```python
from build123d import *

# Parameters (mm, degrees)
EXTRUDE_1_DEPTH     = 20
CHAMFER_1_SIZE      = 10
CUT_EXTRUDE_1_DEPTH = 15
SKETCH_3_R          = 15
CUT_EXTRUDE_2_DEPTH = 20
SKETCH_4_R          = 2.25
SKETCH_4_R_2        = 10
CUT_EXTRUDE_3_DEPTH = 20
SKETCH_5_R          = 4
EXTRUDE_3_DEPTH     = 5
FILLET_1_R          = 5
SKETCH_6_R          = 1
CUT_EXTRUDE_4_DEPTH = 10
FILLET_2_R          = 5
CUT_EXTRUDE_5_REACH = 22
EXTRUDE_4_DEPTH     = 13
CUT_EXTRUDE_6_DEPTH = 5


with BuildPart() as part:
    # 스케치1 → 보스-돌출1 (new body)
    with BuildSketch(Plane.XY):
        with BuildLine():
            Line((0, 35), (40, 35))
            ThreePointArc((40, 35), (57.364817767, 36.519224699), (74.202014333, 41.030737921))
            Line((74.202014333, 41.030737921), (83.59894054, 44.450939355))
            ThreePointArc((83.59894054, 44.450939355), (128.458887284, 23.532402644), (107.540350573, -21.3275441))
            Line((107.540350573, -21.3275441), (98.143424365, -24.747745534))
            ThreePointArc((98.143424365, -24.747745534), (69.520190203, -32.417318012), (40, -35))
            Line((40, -35), (0, -35))
            ThreePointArc((0, -35), (-35, 0), (0, 35))
        make_face()
    extrude(amount=EXTRUDE_1_DEPTH)

    # 모따기1
    chamfer_1_edges = [part.edges().sort_by_distance(p)[0] for p in [
        (128.458887284, 23.532402644, 20),
        (78.900477436, 42.740838638, 20),
        (57.364817767, 36.519224699, 20),
        (20, 35, 20),
        (-35, 0, 20),
        (20, -35, 20),
        (69.520190203, -32.417318012, 20),
        (102.841887469, -23.037644817, 20),
    ]]
    chamfer(chamfer_1_edges, length=CHAMFER_1_SIZE)

    # 스케치2 → 컷-돌출1 (cut)
    with BuildSketch(Plane.XY.offset(20)):
        with BuildLine():
            Line((40, 25), (0, 25))
            ThreePointArc((0, 25), (-25, 0), (0, -25))
            Line((0, -25), (40, -25))
            ThreePointArc((40, -25), (67.783708427, -22.569240482), (94.723222932, -15.350819326))
            Line((94.723222932, -15.350819326), (104.12014914, -11.930617892))
            ThreePointArc((104.12014914, -11.930617892), (119.061961076, 20.11220121), (87.019141974, 35.054013147))
            Line((87.019141974, 35.054013147), (77.622215766, 31.633811714))
            ThreePointArc((77.622215766, 31.633811714), (59.101299543, 26.671147169), (40, 25))
        make_face()
    extrude(amount=-CUT_EXTRUDE_1_DEPTH, mode=Mode.SUBTRACT)

    # 스케치3 → 컷-돌출2 (cut)
    with BuildSketch(Plane.XY.offset(5)):
        with Locations((95.569645557, 11.561697627)):
            Circle(SKETCH_3_R)
    extrude(amount=-CUT_EXTRUDE_2_DEPTH, mode=Mode.SUBTRACT)

    # 스케치4 → 컷-돌출3 (cut)
    with BuildSketch(Plane.XY.offset(5)):
        with Locations((-10.606601718, 10.606601718)):
            Circle(SKETCH_4_R)
        with Locations((10.606601718, 10.606601718)):
            Circle(SKETCH_4_R)
        with Locations((10.606601718, -10.606601718)):
            Circle(SKETCH_4_R)
        with Locations((-10.606601718, -10.606601718)):
            Circle(SKETCH_4_R)
        Circle(SKETCH_4_R_2)
    extrude(amount=-CUT_EXTRUDE_3_DEPTH, mode=Mode.SUBTRACT)

    # 스케치5 → 보스-돌출3 (add)
    with BuildSketch(Plane.XY.offset(5)):
        with Locations((-22, 0)):
            Circle(SKETCH_5_R)
        with Locations((116.242883214, 19.08614078)):
            Circle(SKETCH_5_R)
        with Locations((59.622244076, 23.71672391)):
            Circle(SKETCH_5_R)
        with Locations((67.262763894, -19.614817223)):
            Circle(SKETCH_5_R)
    extrude(amount=EXTRUDE_3_DEPTH)

    # 필렛1
    fillet_1_edges = [part.edges().sort_by_distance(p)[0] for p in [
        (-24.840909091, -2.81588983, 7.5),
        (-24.840909091, 2.81588983, 7.5),
        (117.94937348, 22.703859809, 7.5),
        (119.875555567, 17.41171802, 7.5),
        (61.666476802, 27.154908396, 7.5),
        (56.525365318, 26.248391731, 7.5),
        (70.410078123, -22.083503744, 7.5),
        (65.149596455, -23.011068594, 7.5),
    ]]
    fillet(fillet_1_edges, radius=FILLET_1_R)

    # 스케치6 → 컷-돌출4 (cut)
    with BuildSketch(Plane.XY.offset(10)):
        with Locations((59.622244076, 23.71672391)):
            Circle(SKETCH_6_R)
        with Locations((67.262763894, -19.614817223)):
            Circle(SKETCH_6_R)
        with Locations((-22, 0)):
            Circle(SKETCH_6_R)
        with Locations((116.242883214, 19.08614078)):
            Circle(SKETCH_6_R)
    extrude(amount=-CUT_EXTRUDE_4_DEPTH, mode=Mode.SUBTRACT)

    # 필렛2
    fillet_2_edges = [part.edges().sort_by_distance(p)[0] for p in [
        (128.458887284, 23.532402644, 10),
        (78.900477436, 42.740838638, 10),
        (102.841887469, -23.037644817, 10),
        (57.364817767, 36.519224699, 10),
        (69.520190203, -32.417318012, 10),
        (20, 35, 10),
        (20, -35, 10),
        (-35, 0, 10),
    ]]
    fillet(fillet_2_edges, radius=FILLET_2_R)

    # 스케치8 → 컷-돌출5 (cut, up to next)
    with BuildSketch(Plane(origin=(0, 0, 0), x_dir=(-1, 0, 0), z_dir=(0, 0, -1)), mode=Mode.PRIVATE) as cut_extrude_5_sk1:
        with BuildLine():
            ThreePointArc((-79.499955315, -7.589413451), (-72.077330037, 3.011194044), (-70.949451732, 15.902902069))
            ThreePointArc((-70.949451732, 15.902902069), (-73.845591558, 17.930801007), (-75.873490497, 15.03466118))
            ThreePointArc((-75.873490497, 15.03466118), (-76.775793141, 4.721294761), (-82.713893363, -3.759191235))
            ThreePointArc((-82.713893363, -3.759191235), (-83.022035447, -7.281271367), (-79.499955315, -7.589413451))
        make_face()
    cut_extrude_5_tool1 = extrude(cut_extrude_5_sk1.sketch, amount=-CUT_EXTRUDE_5_REACH, mode=Mode.PRIVATE) & part.part
    add(cut_extrude_5_tool1.solids().sort_by_distance((75.648018, 4.310818, 0))[0], mode=Mode.SUBTRACT)

    # 스케치9 → 보스-돌출4 (add)
    with BuildSketch(Plane(origin=(0, 0, 20), x_dir=(-1, 0, 0), z_dir=(0, 0, -1))):
        with BuildLine():
            Line((-107.540350573, -21.3275441), (-98.143424365, -24.747745534))
            ThreePointArc((-98.143424365, -24.747745534), (-69.520190203, -32.417318012), (-40, -35))
            Line((-40, -35), (0, -35))
            ThreePointArc((0, -35), (35, 0), (0, 35))
            Line((0, 35), (-40, 35))
            ThreePointArc((-40, 35), (-57.364817767, 36.519224699), (-74.202014333, 41.030737921))
            Line((-74.202014333, 41.030737921), (-83.59894054, 44.450939355))
            ThreePointArc((-83.59894054, 44.450939355), (-128.458887284, 23.532402644), (-107.540350573, -21.3275441))
        make_face()
        with BuildLine():
            Line((-104.12014914, -11.930617892), (-94.723222932, -15.350819326))
            ThreePointArc((-94.723222932, -15.350819326), (-67.783708427, -22.569240482), (-40, -25))
            Line((-40, -25), (0, -25))
            ThreePointArc((0, -25), (13.589095993, -20.984195722), (22.8125, -10.226917607))
            ThreePointArc((22.8125, -10.226917607), (25, 0), (22.8125, 10.226917607))
            ThreePointArc((22.8125, 10.226917607), (13.589095993, 20.984195722), (0, 25))
            Line((0, 25), (-40, 25))
            ThreePointArc((-40, 25), (-59.101299543, 26.671147169), (-77.622215766, 31.633811714))
            Line((-77.622215766, 31.633811714), (-87.019141974, 35.054013147))
            ThreePointArc((-87.019141974, 35.054013147), (-119.061961076, 20.11220121), (-104.12014914, -11.930617892))
        make_face(mode=Mode.SUBTRACT)
    extrude(amount=EXTRUDE_4_DEPTH)

    # 스케치10 → 컷-돌출6 (cut)
    with BuildSketch(Plane(origin=(0, 0, 20), x_dir=(-1, 0, 0), z_dir=(0, 0, -1))):
        with BuildLine():
            Line((-74.202014333, 41.030737921), (-83.59894054, 44.450939355))
            ThreePointArc((-83.59894054, 44.450939355), (-128.458887284, 23.532402644), (-107.540350573, -21.3275441))
            Line((-107.540350573, -21.3275441), (-98.143424365, -24.747745534))
            ThreePointArc((-98.143424365, -24.747745534), (-69.520190203, -32.417318012), (-40, -35))
            Line((-40, -35), (0, -35))
            ThreePointArc((0, -35), (35, 0), (0, 35))
            Line((0, 35), (-40, 35))
            ThreePointArc((-40, 35), (-57.364817767, 36.519224699), (-74.202014333, 41.030737921))
        make_face()
        with BuildLine():
            Line((-40, -25), (0, -25))
            ThreePointArc((0, -25), (25, 0), (0, 25))
            Line((0, 25), (-40, 25))
            ThreePointArc((-40, 25), (-59.101299543, 26.671147169), (-77.622215766, 31.633811714))
            Line((-77.622215766, 31.633811714), (-87.019141974, 35.054013147))
            ThreePointArc((-87.019141974, 35.054013147), (-119.061961076, 20.11220121), (-104.12014914, -11.930617892))
            Line((-104.12014914, -11.930617892), (-94.723222932, -15.350819326))
            ThreePointArc((-94.723222932, -15.350819326), (-67.783708427, -22.569240482), (-40, -25))
        make_face(mode=Mode.SUBTRACT)
    extrude(amount=CUT_EXTRUDE_6_DEPTH, mode=Mode.SUBTRACT)


solid = part.part
```
Verification items for the finished model (mm, model axes). A direction names the side the tool comes from. Round coordinates to 2 decimals unless told otherwise and drop trailing zeros. Order: outer loops, then holes, each group sorted by start corner. A loop starts at its lowest first (then second) coordinate and runs counter-clockwise, first axis right, second up. Notation, with made-up numbers: (77.5, 26.25) -> (81.5, 26.25) arc R21 cw to (81.5, 54.25) -> close; hole circle Ø8 at (4.25, -28.5). An arc over 180 degrees is marked (long way). Put each result on its own line as item: value. Start each with the question number.
(1) Section check A-A (z = 12.5). Enter the section's corners in (x, y).
(2) Material ranges on line 1 along Y through (x, z) = (23, 12.25); line 2 along Z through (x, y) = (109, 23); line 3 along Z through (x, y) = (66, -21), recorded low to high.
(3) Section check B-B (y = -6). State how many separate pieces and enclosed holes the cut face has, then the cut area to 3 significant figures.
(4) Section check C-C (y = -28). Enter the section's corners in (x, z).
(5) Draft check along Z on faces 4 (the face through (-9.397, 12.504, 2.535)), 5 (the face through (48, 6, 5)). Enter one of: +Z half, -Z half, draft (parallel to the pull), parting line (faces both ways), or undercut.
(6) Depth check by flat-ended pin: pin 1 Ø1.8 at (x, y) = (116.24, 19.09) entering from -Z; pin 2 Ø1.5 at (y, z) = (18, 3) entering from +X; pin 3 Ø1.5 at (x, y) = (81.5, 24) entering from +Z; pin 4 Ø7.5 at (x, z) = (18, 5.5) entering from +Y. Enter the tip coordinate at first touch or a pass-through.
(7) Tool access check on faces 1 (the face through (60.24, 19.765, 7.465)), 2 (the face through (72.14, 2.84, 2.46)), 3 (the face through (78.835, 42.717, 7.605)). Record the directions out of +Z, -Z, +X, -X, +Y, -Y that give a thin tool (end or side, any length) a straight path to the whole face; none if there is none.
Completed:
1. outline: (0, -35) -> (40, -35) arc R170 ccw to (98.14, -24.75) -> (107.54, -21.33) arc R35 ccw to (83.6, 44.45) -> (74.2, 41.03) arc R100 cw to (40, 35) -> (0, 35) arc R35 ccw to start; hole (0, -25) -> (40, -25) arc R160 ccw to (94.72, -15.35) -> (104.12, -11.93) arc R25 ccw to (87.02, 35.05) -> (77.62, 31.63) arc R110 cw to (40, 25) -> (0, 25) arc R25 ccw to start
2. line 1: y = -35 to -25, 25 to 35
2. line 2: z = 0 to 5
2. line 3: z = 0 to 10
3. separate pieces: 3
3. enclosed holes: 0
3. area: 927 mm2
4. outline: (-21, 0) -> (88.28, 0) -> (88.28, 15) -> (-21, 15) -> close
5. face 4: draft
5. face 5: +Z half
6. pin 1: passes through
6. pin 2: stops at x = 130.1
6. pin 3: stops at z = 5
6. pin 4: stops at y = 35
7. face 1: +Z
7. face 2: +Z, -Z
7. face 3: +Z, -Z, -X, +Y
